Can you work these out from the drawing? Everything is in mm from the part's minimum corner. Round coordinates to 2 decimals unless told otherwise and drop trailing zeros. Write each loop counter-clockwise with the first axis right and the second up, starting at its lowest first coordinate (ties: lowest second). Pieces come first, ordered by that corner, then holes. Notation, with made-up numbers: (-27.75, 41) -> (14.25, 41) arc R12 ccw to (14.25, 45) -> close; hole circle Ø7 at (65.25, 74). An arc over 180 degrees is marked (long way). Put each result on its own line as item: value. Start each with the question number.
1. Suppose I cut it at B-B (y = 90). Please give me the cut outline in (x, z).
2. Suppose I cut it at C-C (z = 90.5). Please give me the cut outline in (x, y), then the cut area to 3 significant figures.
3. We'd pull the mould along Z, two halves only. Please class the marked faces 1, 2, 3 and 4: +Z half, -Z half, draft (parallel to the pull), parting line (faces both ways), or undercut.
4. Suppose I cut it at A-A (x = 85). Please give me the cut outline in (y, z).
5. I need wall thicknesses on probe 1 along X at (y, z) = (57, 66); probe 2 along Z at (x, y) = (115, 21). Which ranges of each line are inside material? Lowest first, please. Write a range as from..to.
6. Suppose I cut it at D-D (y = 42.5). Please give me the cut outline in (x, z).
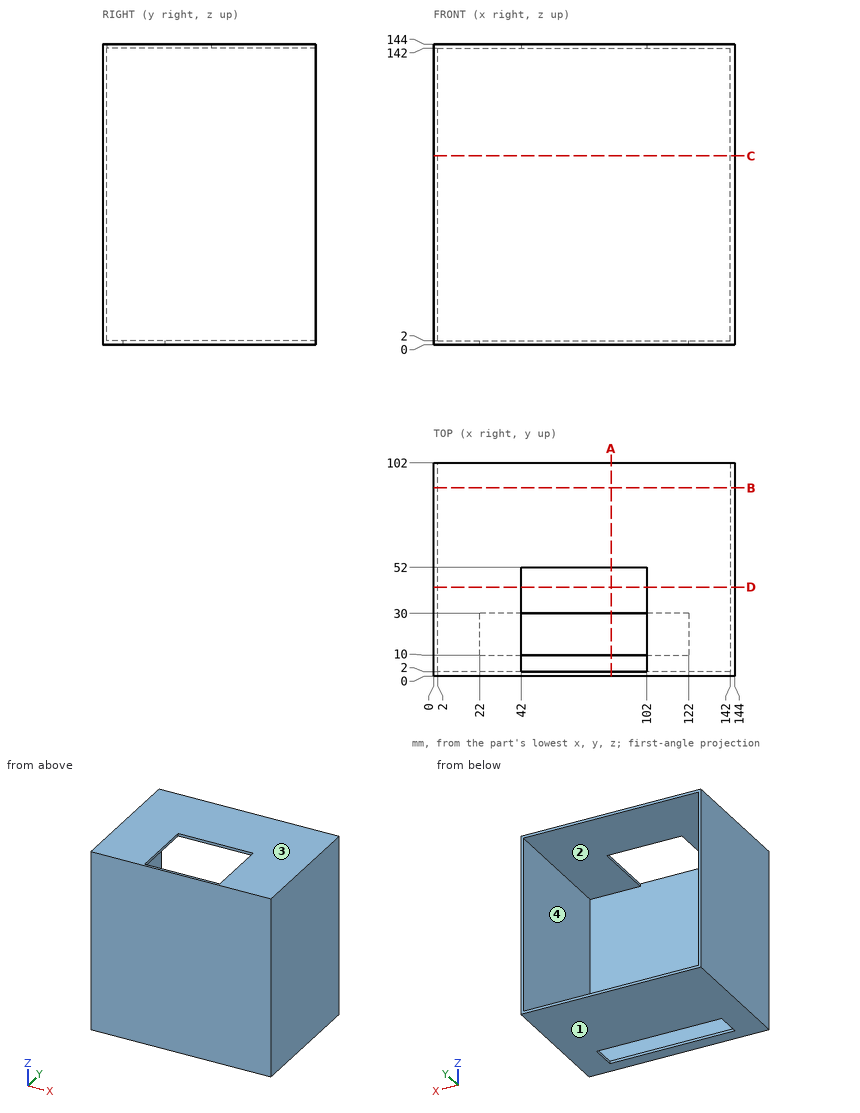
Verdict:
1. outline: (0, 0) -> (144, 0) -> (144, 144) -> (0, 144) -> close; hole (2, 2) -> (142, 2) -> (142, 142) -> (2, 142) -> close
2. outline: (0, 0) -> (144, 0) -> (144, 102) -> (142, 102) -> (142, 2) -> (2, 2) -> (2, 102) -> (0, 102) -> close
2. area: 688 mm^2
3. face 1: -Z half
3. face 2: undercut
3. face 3: +Z half
3. face 4: undercut
4. outline: (0, 0) -> (10, 0) -> (10, 2) -> (2, 2) -> (2, 144) -> (0, 144) -> close; (30, 0) -> (102, 0) -> (102, 2) -> (30, 2) -> close; (52, 142) -> (102, 142) -> (102, 144) -> (52, 144) -> close
5. probe 1: x = 0..2, 142..144
5. probe 2: z = 142..144
6. outline: (0, 0) -> (144, 0) -> (144, 144) -> (102, 144) -> (102, 142) -> (142, 142) -> (142, 2) -> (2, 2) -> (2, 142) -> (42, 142) -> (42, 144) -> (0, 144) -> close
